Part model, mm, in its own coordinate system. Face numbers are marked on the shaded views. A direction names the side the tool comes from. Coordinates: 2 decimals unless noted, no trailing zeros. Write each loop counter-clockwise with the first axis right and the second up, starting at its lowest first coordinate (ties: lowest second). Pieces come first, ordered by that corner, then holes. Notation, with made-up numbers: (81, -25.5) - (85, -25.5) arc R6 cw to (85, -21.5) - close; hole circle Ø7 at (2.5, 55). An arc over 180 degrees is marked (long way). Use a Markdown table: item, result.
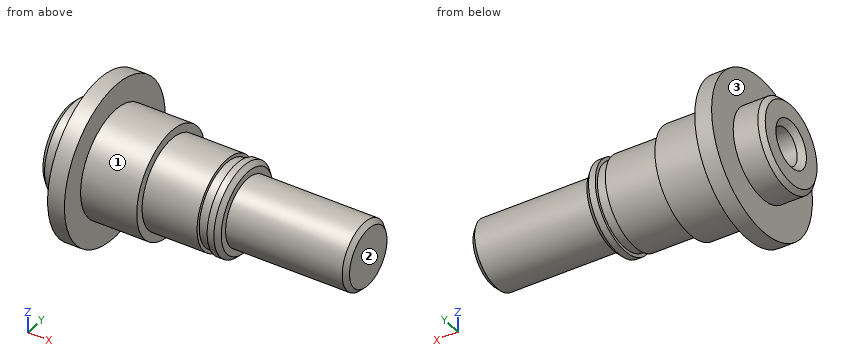
Autodesk Inventor part; units mm, degrees
ref_plane "Work Plane4" through (26.7, 0, 0) normal (1, 0, 0) x (0, 0, -1)
ref_plane "YZ Plane" through (0, 0, 0) normal (1, 0, 0) x (0, 1, 0)
ref_plane "XZ Plane" through (0, 0, 0) normal (0, 1, 0) x (-1, 0, 0)
sketch "Sketch1" plane through (0, 0, 0) normal (0, 0, 1) x (1, 0, 0)
  line L0 (15.9, 4) -> (15.9, 3)
  line L1 (15.9, 3) -> (26.7, 3)
  line L2 (26.7, 3) -> (26.7, 0)
  line L3 (26.7, 0) -> (0, 0)
  line L4 (0, 0) -> (0, 4)
  line L5 (4.1, 4.75) -> (9.1, 4.75)
  line L6 (9.1, 4.75) -> (9.1, 4)
  line L7 (0, 4) -> (2.6, 4)
  line L8 (14, 4) -> (14, 3.7)
  line L9 (14, 3.7) -> (14.9, 3.7)
  line L10 (14.9, 3.7) -> (14.9, 4)
  line L11 (9.1, 4) -> (14, 4)
  line L12 (14.9, 4) -> (15.9, 4)
  line L13 (14.1, 4) -> (14.1, 0) construction
  line L14 (4.1, 4.75) -> (4.1, 0) construction
  line L15 (16.7, 3) -> (16.7, 0) construction
  line L16 (18.2, 3) -> (18.2, 0) construction
  line L17 (2.6, 4) -> (2.6, 7)
  line L18 (2.6, 7) -> (4.1, 7)
  line L19 (4.1, 7) -> (4.1, 4.75)
  line L20 (9.1, 4) -> (9.1, 0) construction
  line L21 (6.1, 4.75) -> (6.1, 0) construction
  dimension "d0" = 6
  dimension "d2" = 9.5
  dimension "d3" = 8
  dimension "d7" = 0.9
  dimension "d8" = 7.4
  dimension "d9" = 1
  dimension "Cover_MountingPlate_Thickness" = 1.5
  dimension "d23" = 0.8
  dimension "MountingPlate_MEnc_Distance" = 14.1
  dimension "d25" = 8.5
  dimension "d29" = 14
  dimension "d31" = 1.5
  dimension "d32" = 2.6
  dimension "d33" = 0.1
  dimension "d34" = 5
  dimension "d35" = 8
  dimension "d36" = 2
revolve "Revolution1" add sketch "Sketch1" angle 360 about axis through (26.7, 0, 0) along (-1, 0, 0)
chamfer "Chamfer1" distance 0.4 angle 45 3 edges at (0, -4, 0) (26.7, -3, 0) (15.9, -4, 0)
ref_plane "Work Plane4" through (26.7, 0, 0) normal (1, 0, 0) x (0, 0, -1)
ref_plane "Work Plane3" through (18.2, 0, 0) normal (1, 0, 0) x (0, 0, -1)
sketch "Sketch2" plane through (0, 0, 0) normal (-1, 0, 0) x (0, 0, 1)
  point P0 (0, 0)
  point P1 (0, 0)
hole "Hole1" at (0, 0, 0) direction (1, 0, 0) diameter 3.242 depth 6 tip angle 118
chamfer "Chamfer2" distance 0.5 angle 45 1 edges at (0, 0, -1.621)
ref_plane "Work Plane2" through (16.7, 0, 0) normal (1, 0, 0) x (0, 0, -1)
equation "\"d35\" = ShaftFixation_UpperLower_Height"
equation "\"d36\" = BasePlate_UpperLowerConnector_Height"
equation "\"d18\" = d23"
equation "\"d19\" = Cover_MountingPlate_Thickness"
equation "\"d20\" = d25"
properties part number "UpperLowerArm_JointShaft" material "Aluminum 6061"
Item 1: Band-saw the part on A-A, the plane x = 21.5. Give the cut face in (y, z), then the cut area to 3 significant figures.
From the geometry:
| item | result |
|---|---|
| outline | circle Ø6 at (0, 0) |
| area | 28.3 mm^2 |
Item 2: Drill centre lines: probe 1 along Z at (x, y) = (4.7, 0); probe 2 along Z at (x, y) = (3.5, 0). Where is each one in solid material? Low to high.
From the geometry:
| item | result |
|---|---|
| probe 1 | -4.75 to -1.62, 1.62 to 4.75 |
| probe 2 | -7 to -1.62, 1.62 to 7 |
Item 3: Band-saw the part on B-B, the plane z = 6. Give the cut face in (x, y), then the cut area to 3 significant figures.
From the geometry:
| item | result |
|---|---|
| outline | (2.6, -3.61) - (4.1, -3.61) - (4.1, 3.61) - (2.6, 3.61) - close |
| area | 10.8 mm^2 |
Item 4: Which spindle directions (+Z, -Z, +X, -X, +Y, -Y) get a long thin tool onto all of the face, cutting with end or side? Do the marked faces 1, 2 and 3. Say none if no direction does.
From the geometry:
| item | result |
|---|---|
| face 1 | +X |
| face 2 | +Z, -Z, +X, +Y, -Y |
| face 3 | -X |
Item 5: Drop flat-ended pins along their axis: P1, Ø3, axis at x = 6, y = 1, coming from the +Z side; P2, Ø6, axis at x = 18, z = 5.5, coming from the +Y side; P3, Ø4, axis at x = 21, y = 4.5, coming from the -Z side. Give the stop position or say it passes through.
From the geometry:
| item | result |
|---|---|
| P1 | z = 4.75 |
| P2 | y = 1.66 |
| P3 | z = -1.66 |
Item 6: Band-saw the part on D-D, the plane x = 10.5. Give the cut face in (y, z).
From the geometry:
| item | result |
|---|---|
| outline | circle Ø8 at (0, 0) |
Item 7: Band-saw the part on C-C, the plane y = 5.75. Give the cut face in (x, z), then the cut area to 3 significant figures.
From the geometry:
| item | result |
|---|---|
| outline | (2.6, -3.99) - (4.1, -3.99) - (4.1, 3.99) - (2.6, 3.99) - close |
| area | 12.0 mm^2 |
